The drawing under review shows one solid part. Ordinate dimensions are in mm from its lowest x, y, z. A direction names the side the tool comes from. Coordinates: 2 decimals unless noted, no trailing zeros. Write each loop counter-clockwise with the first axis right and the second up, starting at its lowest first coordinate (ties: lowest second). Pieces come first, ordered by that corner, then holes. Notation, with made-up numbers: (-14.5, -5) - (36.5, -5) arc R18 cw to (36.5, 10) - close; hole circle Ø3 at (32.5, 15). An arc over 180 degrees is marked (long way). Use a Markdown table: item, result.
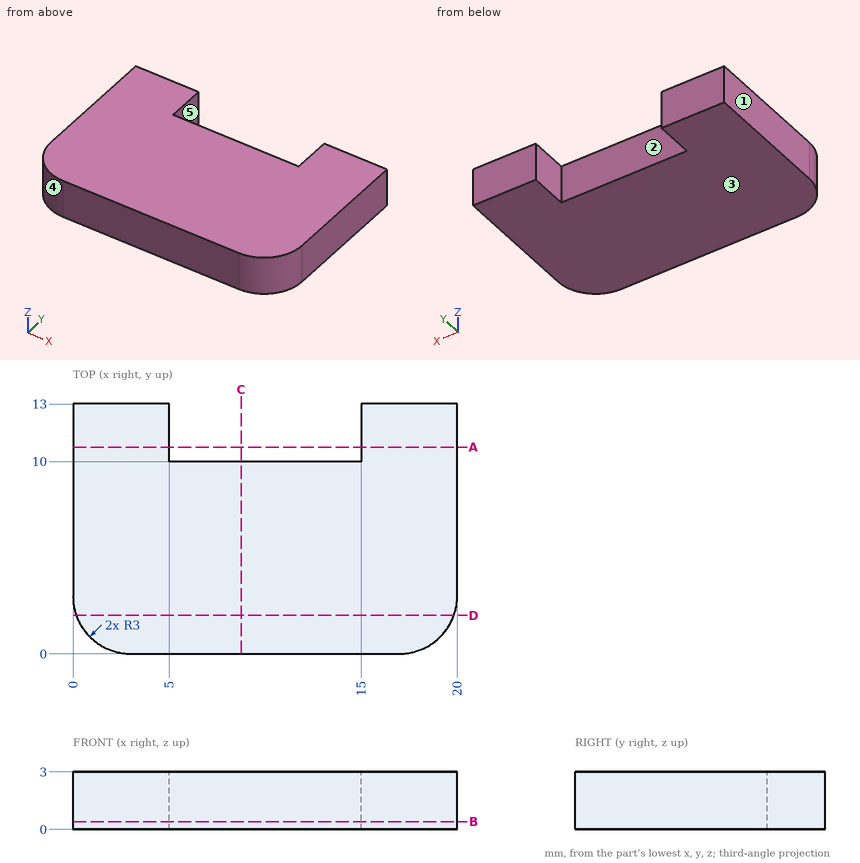
(1) Take a section at B-B on z = 0.4. Write out the cut boundary in (x, y), and give its area (3 significant figures).
Determined:
| item | result |
|---|---|
| outline | (0, 3) arc R3 ccw to (3, 0) - (17, 0) arc R3 ccw to (20, 3) - (20, 13) - (15, 13) - (15, 10) - (5, 10) - (5, 13) - (0, 13) - close |
| area | 226 mm2 |
(2) Take a section at A-A on y = 10.75. Write out the cut boundary in (x, z).
Determined:
| item | result |
|---|---|
| outline | (0, 0) - (5, 0) - (5, 3) - (0, 3) - close; (15, 0) - (20, 0) - (20, 3) - (15, 3) - close |
(3) Draft analysis for pull direction X (two halves, no side actions). For the marked faces 3, 4 and 5, state which applies: +X half, -X half, draft (parallel to the pull), parting line (faces both ways), or undercut.
Determined:
| item | result |
|---|---|
| face 3 | draft |
| face 4 | -X half |
| face 5 | undercut |
(4) Machinability: for the marked faces 1 and 2, which of the approach directions +Z, -Z, +X, -X, +Y, -Y give a long, thin tool a straight path to every point of the face, cutting with its end or side? Answer none if there is none.
Determined:
| item | result |
|---|---|
| face 1 | +Z, -Z, -X, +Y, -Y |
| face 2 | +Z, -Z, +Y |
(5) Take a section at D-D on y = 2. Write out the cut boundary in (x, z), and give its area (3 significant figures).
Determined:
| item | result |
|---|---|
| outline | (0.17, 0) - (19.83, 0) - (19.83, 3) - (0.17, 3) - close |
| area | 59.0 mm2 |
(6) Take a section at C-C on x = 8.75. Write out the cut boundary in (y, z).
Determined:
| item | result |
|---|---|
| outline | (0, 0) - (10, 0) - (10, 3) - (0, 3) - close |
(7) For L1, parallel to X at y = 10.5, z = 2.8; L2, parallel to Y at x = 5.5, z = 0.75; L3, parallel to Y at x = 18.25, z = 2.25, list the stretches that pass through material, from the lowest coordinate up. Write a range as from..to.
Determined:
| item | result |
|---|---|
| L1 | 0..5, 15..20 |
| L2 | 0..10 |
| L3 | 0.27..13 |
(8) For pin 1 (1.5 mm diameter, centred on x = 7.5, z = 1, fed in from +Y); pin 2 (1.5 mm diameter, centred on y = 2, z = 1.5, fed in from +X), all flat-tipped, find the tip position at first contact; note any pin that passes through.
Determined:
| item | result |
|---|---|
| pin 1 | y = 10 |
| pin 2 | x = 19.99 |
